Work out the finished part from the listing and answer in its coordinate system (mm). A direction names the side the tool comes from. Round coordinates to 2 decimals unless told otherwise and drop trailing zeros. Order: outer loops, then holes, each group sorted by start corner. A loop starts at its lowest first (then second) coordinate and runs counter-clockwise, first axis right, second up. Notation, with made-up numbers: (44, -25.5) -> (59, -25.5) arc R23 cw to (59, 1.5) -> close; hole circle Ø2 at (64, 3). An arc over 180 degrees is marked (long way). Use one line per item in the form item = value.
```python
from build123d import *

# Parameters (mm, degrees)
BOSS_EXTRUDE1_DEPTH = 28.5
SKETCH3_R           = 2
CUT_EXTRUDE1_DEPTH  = 29.81405906844782
SKETCH4_W           = 5.000000000000001
SKETCH4_H           = 6
SKETCH4_W_2         = 6
SKETCH4_H_2         = 5
BOSS_EXTRUDE2_DEPTH = 5
FILLET1_R           = 10
FILLET3_R           = 5
FILLET4_R           = 5
FILLET5_R           = 2
CUT_EXTRUDE2_START  = -4
SKETCH5_R           = 2.5
CUT_EXTRUDE2_DEPTH  = 4
CUT_EXTRUDE3_START  = -8
SKETCH6_R           = 2.5
CUT_EXTRUDE3_DEPTH  = 4
FILLET6_R           = 1


# Some blends are built 0.0001 mm under size
with BuildPart() as part:
    # Sketch2 → Boss-Extrude1 (new body)
    with BuildSketch(Plane(origin=(0, 0, 0), x_dir=(1, 0, 0), z_dir=(0, 1, 0))):
        Polygon((-3.000000000000001, 3), (2.999999999999999, 3), (3, -3), (-3, -3), align=None)
    extrude(amount=BOSS_EXTRUDE1_DEPTH)

    # Sketch3 → Cut-Extrude1 (cut, through all)
    with BuildSketch(Plane.XZ):
        with Locations(Location((0, 0, 0), (0, 0, 270))):
            Circle(SKETCH3_R)
    extrude(amount=-CUT_EXTRUDE1_DEPTH, mode=Mode.SUBTRACT)

    # Sketch4 → Boss-Extrude2 (add)
    with BuildSketch(Plane.XZ):
        with Locations((5.5, 0)):
            Rectangle(SKETCH4_W, SKETCH4_H)
        with Locations((0, 5.5)):
            Rectangle(SKETCH4_W_2, SKETCH4_H_2)
    extrude(amount=-BOSS_EXTRUDE2_DEPTH)

    # Fillet1
    # the kernel refuses this fillet: 10 mm, written as the material it adds along each edge
    with BuildSketch(Plane(origin=(3, 0, 3), x_dir=(3.6e-16, 0, 1), z_dir=(0, 1, 0))) as fillet1_piece_1:
        with BuildLine():
            CenterArc((9.11437827766148, 9.114378277661475), FILLET1_R, 204.29518894536457, 41.4096221092708)
            Line((1.78e-15, 5), (0, 0))
            Line((0, 0), (5, 0))
        make_face()
    extrude(amount=5)

    # Fillet3
    # the kernel refuses this fillet: 5 mm, written as the material it adds along each edge
    with BuildSketch(Plane(origin=(3, 5, 3), x_dir=(0, 0, 1), z_dir=(-1, 0, 0))) as fillet3_piece_1:
        with BuildLine():
            CenterArc((FILLET3_R, FILLET3_R), FILLET3_R, 180, 90)
            Line((-8.9e-16, FILLET3_R), (0, 0))
            Line((0, 0), (FILLET3_R, 0))
        make_face()
    extrude(amount=6)
    with BuildSketch(Plane(origin=(2.999999999999999, 5, 3), x_dir=(1, 0, 0), z_dir=(0, 0, -1))) as fillet3_piece_2:
        with BuildLine():
            CenterArc((FILLET3_R, -FILLET3_R), FILLET3_R, 90, 90)
            Line((-8.9e-16, -FILLET3_R), (0, 0))
            Line((0, 0), (FILLET3_R, 0))
        make_face()
    extrude(amount=6)
    with BuildSketch(Plane(origin=(15.5, 5, 3), x_dir=(0, 0, 1), z_dir=(-1, 0, 0))) as fillet3_piece_3a_section:
        with BuildLine():
            CenterArc((FILLET3_R, FILLET3_R), FILLET3_R, 180, 90)
            Line((-8.9e-16, FILLET3_R), (0, 0))
            Line((0, 0), (FILLET3_R, 0))
        make_face()
    fillet3_piece_3a = extrude(amount=18.5, mode=Mode.PRIVATE)
    fillet3_piece_3a = fillet3_piece_3a - Plane(origin=(12.114378277661, 5, 12.114378277661), x_dir=(0, 0, 1), z_dir=(0, -1, 0)) * Cylinder(10, 57, mode=Mode.PRIVATE)
    fillet3_piece_3a = split(fillet3_piece_3a, bisect_by=Plane(origin=(8, 5, 3), z_dir=(-1, 0, 0)), keep=Keep.TOP, mode=Mode.PRIVATE)
    fillet3_piece_3a = split(fillet3_piece_3a, bisect_by=Plane(origin=(3, 5, 3.0000000000000018), z_dir=(1, 0, -1.5e-16)), keep=Keep.TOP, mode=Mode.PRIVATE)
    with BuildSketch(Plane(origin=(2.999999999999999, 5, 15.5), x_dir=(1, 0, 0), z_dir=(0, 0, -1))) as fillet3_piece_3b_section:
        with BuildLine():
            CenterArc((FILLET3_R, -FILLET3_R), FILLET3_R, 90, 90)
            Line((-8.9e-16, -FILLET3_R), (0, 0))
            Line((0, 0), (FILLET3_R, 0))
        make_face()
    fillet3_piece_3b = extrude(amount=18.5, mode=Mode.PRIVATE)
    fillet3_piece_3b = fillet3_piece_3b - Plane(origin=(12.114378277661, 5, 12.114378277661), x_dir=(0, 0, 1), z_dir=(0, -1, 0)) * Cylinder(10, 57, mode=Mode.PRIVATE)
    fillet3_piece_3b = split(fillet3_piece_3b, bisect_by=Plane(origin=(2.999999999999999, 5, 8), z_dir=(0, 0, -1)), keep=Keep.TOP, mode=Mode.PRIVATE)
    fillet3_piece_3b = split(fillet3_piece_3b, bisect_by=Plane(origin=(2.999999999999999, 5, 3), z_dir=(0, 0, 1)), keep=Keep.TOP, mode=Mode.PRIVATE)
    fillet3_piece_3 = fillet3_piece_3a & fillet3_piece_3b
    add(fillet3_piece_3)

    # Fillet4
    fillet4_edges = [part.edges().sort_by_distance(p)[0] for p in [
        (8, 2.5, 3),
        (8, 5, 0),
        (3, 2.5, 8),
        (0, 5, 8),
    ]]
    fillet(fillet4_edges, radius=FILLET4_R)

    # Mirror1: part across plane


with BuildPart() as part_1:
    add(part.part)
    add(part.part.mirror(Plane.ZX.offset(28.5)))

    # Fillet5
    fillet5_edges = [part_1.edges().sort_by_distance(p)[0] for p in [
        (-3.000000000000001, 28.5, -3),
    ]]
    fillet(fillet5_edges, radius=FILLET5_R)

    # Sketch5 → Cut-Extrude2 (cut)
    with BuildSketch(Plane.XZ.offset(CUT_EXTRUDE2_START)):
        with Locations(Location((0, 0, 0), (0, 0, 270))):
            Circle(SKETCH5_R)
    extrude(amount=-CUT_EXTRUDE2_DEPTH, mode=Mode.SUBTRACT)

    # Sketch6 → Cut-Extrude3 (cut)
    with BuildSketch(Plane(origin=(0, 57, 0), x_dir=(1, 0, 0), z_dir=(0, 1, 0)).offset(CUT_EXTRUDE3_START)):
        with Locations(Location((0, 0, 0), (0, 0, 90))):
            Circle(SKETCH6_R)
    extrude(amount=CUT_EXTRUDE3_DEPTH, mode=Mode.SUBTRACT)

    # Fillet6
    fillet6_edges = [part_1.edges().sort_by_distance(p)[0] for p in [
        (6.1e-16, 57, 2),
        (6.1e-16, 0, 2),
    ]]
    fillet(fillet6_edges, radius=FILLET6_R - 0.0001)  # a hair under: the kernel refuses the full size


solid = part_1.part
```
Item 1: Determine the mould class of faces 1 (the flat face through (3, 57, 3)), 2 (the cylindrical face through (-2, 29, 0)), 3 (the flat face through (3, 28, 0)) for opening direction Y: released by +Y, released by -Y, zero draft, split by the parting line, or undercut.
Findings:
face_1 = released by +Y
face_2 = zero draft
face_3 = undercut
Item 2: The part is cut by section B-B, the plane y = 4.5. Give the vertices of the cut face in (x, z).
Findings:
outline = (-3, -1) arc R2 ccw to (-1, -3) -> (6.87, -3) -> (6.87, 3.36) arc R5 ccw to (6.04, 4.17) arc R10 cw to (4.17, 6.04) arc R5 ccw to (3.36, 6.87) -> (-3, 6.87) -> close; hole circle Ø5 at (0, 0)
Item 3: For faces 4 (the flat face through (-2, 49, 1)), 5 (the cylindrical face through (-2, 55, 0)), 6 (the flat face through (0, 29, 3)), determine the directions among +Z, -Z, +X, -X, +Y, -Y from which every point of the face is accessible in a straight line to the end or side of a thin tool.
Findings:
face_4 = none
face_5 = +Y, -Y
face_6 = +Z, +X, -X
Item 4: Flat-ended cylindrical pins translate along their axes: P1, Ø4, axis at x = -0.5, z = 1, coming from the -Y side; P2, Ø3, axis at y = 47, z = 2.5, coming from the +X side; P3, Ø6.5, axis at x = 0.5, y = 32.5, coming from the +Z side; P4, Ø5, axis at x = 0, z = 0, coming from the -Y side. Find the tip coordinate at first contact, or state that the pin passes through.
Findings:
P1 = 0
P2 = 3.23
P3 = 3
P4 = 0.13
Item 5: The part is cut by section A-A, the plane y = 38. Give the vertices of the cut face in (x, z), and give its area (3 significant figures).
Findings:
outline = (-3, -1) arc R2 ccw to (-1, -3) -> (3, -3) -> (3, 3) -> (-3, 3) -> close; hole circle Ø4 at (0, 0)
area = 22.6 mm^2
Item 6: Consider line 1 along Z through (x, y) = (0, 33); line 2 along Z through (x, y) = (0, 3.25). Determine where each line is inside the solid, lowest interval first.
Findings:
line_1 = -3 to -2, 2 to 3
line_2 = -3 to -2, 2 to 7.62
